Verification items for this drawing (mm, ordinates from the low corner). A direction names the side the tool comes from. Round coordinates to 2 decimals unless told otherwise and drop trailing zeros. Loops run counter-clockwise (first coordinate to the right, second up) from the corner with the lowest first, then second, coordinate; pieces in that order, holes last. Notation, with made-up numbers: (47.5, 56) - (95.5, 56) arc R16 ccw to (95.5, 64) - close; hole circle Ø6 at (79.25, 61.25). An arc over 180 degrees is marked (long way). Use a Markdown table: item, result. Add a question column.
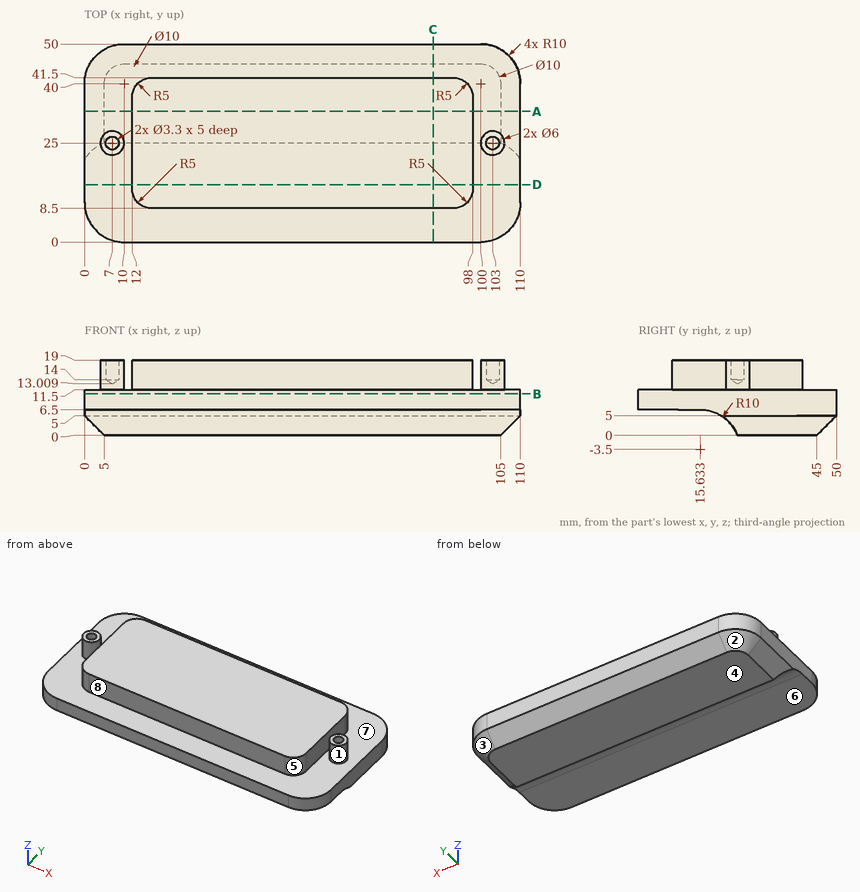
Q1. Release check for a two-part mould opening along X. For the marked faces 1, 2, 3 and 4 record: +X half, -X half, draft (parallel to the pull), parting line (faces both ways), or undercut.
Q2. Section check C-C on x = 88. Record the cut outline in (y, z), plus the area to 3 significant figures.
Q3. Go/stop test with flat-tipped pins: pin 1 Ø8 at (x, y) = (54, 8) entering from -Z; pin 2 Ø8 at (x, z) = (65, 15) entering from -Y; pin 3 Ø8 at (x, z) = (51, 16.5) entering from +Y; pin 4 Ø3.5 at (y, z) = (26.5, 14) entering from +X. Record where each tip stops, or that it passes through.
Q4. Section check B-B on z = 10.5. Record the cut outline in (x, y).
Q5. Set-up check for the marked faces 5, 6, 7 and 8: record each of +Z, -Z, +X, -X, +Y, -Y from which the full face is reachable in a straight line by a thin tool's end or side.
Q6. Section check A-A on y = 33. Record the cut outline in (x, z).
Q7. Section check D-D on y = 14.5. Record the cut outline in (x, z).
Q8. Thickness scan on line 1 along Y through (x, z) = (103, 15.4); line 2 along Z through (x, y) = (82, 12); line 3 along Z through (x, y) = (53, 5.5). Record the ranges inside material, lowest first.
Determined:
| question | item | result |
|---|---|---|
| 1 | face 1 | undercut |
| 1 | face 2 | -X half |
| 1 | face 3 | +X half |
| 1 | face 4 | draft |
| 2 | outline | (0, 6.5) - (15.63, 6.5) arc R10 cw to (25, 0) - (45, 0) - (50, 5) - (50, 11.5) - (41.5, 11.5) - (41.5, 19) - (8.5, 19) - (8.5, 11.5) - (0, 11.5) - close |
| 2 | area | 664 mm² |
| 3 | pin 1 | stops at z = 6.5 |
| 3 | pin 2 | stops at y = 0 |
| 3 | pin 3 | stops at y = 41.5 |
| 3 | pin 4 | stops at x = 106 |
| 4 | outline | (0, 10) arc R10 ccw to (10, 0) - (100, 0) arc R10 ccw to (110, 10) - (110, 40) arc R10 ccw to (100, 50) - (10, 50) arc R10 ccw to (0, 40) - close |
| 5 | face 5 | +Z, +X, -Y |
| 5 | face 6 | -Z, +X, -X, -Y |
| 5 | face 7 | +Z |
| 5 | face 8 | +Z, +X, -X, -Y |
| 6 | outline | (0, 5) - (5, 0) - (105, 0) - (110, 5) - (110, 11.5) - (98, 11.5) - (98, 19) - (12, 19) - (12, 11.5) - (0, 11.5) - close |
| 7 | outline | (0, 6.5) - (110, 6.5) - (110, 11.5) - (98, 11.5) - (98, 19) - (12, 19) - (12, 11.5) - (0, 11.5) - close |
| 8 | line 1 | y = 22 to 23.35, 26.65 to 28 |
| 8 | line 2 | z = 6.5 to 19 |
| 8 | line 3 | z = 6.5 to 11.5 |
